from build123d import *
from OCP.BRepFilletAPI import BRepFilletAPI_MakeChamfer

# Parameters (mm, degrees)
SKETCH1_R           = 11.1125
SKETCH1_R_2         = 3.96875
BOSS_EXTRUDE1_DEPTH = 127
CHAMFER1_SIZE       = 0.762
CHAMFER1_SIZE2      = 0.439940905


with BuildPart() as part:
    # Sketch1 → Boss-Extrude1 (new body)
    with BuildSketch(Plane(origin=(0, 0, 0), x_dir=(0, 0, -1), z_dir=(1, 0, 0))):
        Circle(SKETCH1_R)
        Circle(SKETCH1_R_2, mode=Mode.SUBTRACT)
    extrude(amount=BOSS_EXTRUDE1_DEPTH)

    # Chamfer1: one chamfer whose edges measure the first distance from different faces: ONE call of the kernel's chamfer builder (chamfer() names one face for all edges)
    chamfer1_edges_1 = [part.edges().sort_by_distance(p)[0] for p in [
        (0, 0, 11.1125),
    ]]
    chamfer1_side_1 = [part.faces().sort_by_distance(p)[0] for p in [
        (0, 0, 10.798191036),
    ]]
    chamfer1_edges_2 = [part.edges().sort_by_distance(p)[0] for p in [
        (127, 0, 11.1125),
    ]]
    chamfer1_side_2 = [part.faces().sort_by_distance(p)[0] for p in [
        (63.5, 0, 11.1125),
    ]]
    chamfer1_edges_3 = [part.edges().sort_by_distance(p)[0] for p in [
        (0, 0, 3.96875),
    ]]
    chamfer1_side_3 = [part.faces().sort_by_distance(p)[0] for p in [
        (63.5, 0, 3.96875),
    ]]
    chamfer1_edges_4 = [part.edges().sort_by_distance(p)[0] for p in [
        (127, 0, 3.96875),
    ]]
    chamfer1_side_4 = [part.faces().sort_by_distance(p)[0] for p in [
        (127, 0, 10.798191036),
    ]]
    chamfer1 = BRepFilletAPI_MakeChamfer(part.part.solid().wrapped)
    for e in chamfer1_edges_1:
        chamfer1.Add(CHAMFER1_SIZE, CHAMFER1_SIZE2, e.wrapped, chamfer1_side_1[0].wrapped)  # the first distance lies on this face
    for e in chamfer1_edges_2:
        chamfer1.Add(CHAMFER1_SIZE, CHAMFER1_SIZE2, e.wrapped, chamfer1_side_2[0].wrapped)  # the first distance lies on this face
    for e in chamfer1_edges_3:
        chamfer1.Add(CHAMFER1_SIZE, CHAMFER1_SIZE2, e.wrapped, chamfer1_side_3[0].wrapped)  # the first distance lies on this face
    for e in chamfer1_edges_4:
        chamfer1.Add(CHAMFER1_SIZE, CHAMFER1_SIZE2, e.wrapped, chamfer1_side_4[0].wrapped)  # the first distance lies on this face
    add(Compound.cast(chamfer1.Shape()), mode=Mode.REPLACE)


solid = part.part
Build history of the part. All positions in model axes, mm. Round coordinates to 2 decimals unless told otherwise and drop trailing zeros. Loops run counter-clockwise (first coordinate to the right, second up) from the corner with the lowest first, then second, coordinate; pieces in that order, holes last. Notation, with made-up numbers: (13.5, 28) -> (55.5, 28) arc R20 cw to (55.5, 65) -> close; hole circle Ø2 at (81.25, -16). An arc over 180 degrees is marked (long way). Use CSV: the item, a comma, the result in double quotes. Start each with the question number.
Q1. Mould opens along Z. For faces 1 (the face through (127, -2, -5)), 2 (the face through (62.78, -3.874, 0.86)), 3 (the face through (62.46, 3.34, -10.6)) say: +Z half, -Z half, draft (parallel to the pull), parting line (faces both ways), or undercut.
Q2. Flat gauge pins, fed straight in: pin 1 Ø6 at (x, z) = (40, -7.5) entering from -Y; pin 2 Ø3 at (x, y) = (60, 7.5) entering from -Z; pin 3 Ø1.5 at (x, y) = (22.5, -6.5) entering from -Z. Where does each tip first touch, or does it go through?
Q3. Drill centre lines: L1, parallel to Y at x = 35.5, z = 0; L2, parallel to Z at x = 56, y = -0.75; L3, parallel to Y at x = 26, z = -0.5. Where is each one in solid material? Low to high.
Q4. Saw through at A-A on z = 0. Give the cut face in (x, y), and give its area (3 significant figures).
Q5. Saw through at C-C on x = 96. Give the cut face in (y, z) (1 decimal), and give its area (3 significant figures).
Solutions:
1,face 1,"draft"
1,face 2,"undercut"
1,face 3,"parting line"
2,pin 1,"stops at y = -10.16"
2,pin 2,"stops at z = -9.35"
2,pin 3,"stops at z = -9.51"
3,L1,"y = -11.11 to -3.97, 3.97 to 11.11"
3,L2,"z = -11.09 to -3.9, 3.9 to 11.09"
3,L3,"y = -11.1 to -3.94, 3.94 to 11.1"
4,outline,"(0, -10.35) -> (0.44, -11.11) -> (126.24, -11.11) -> (127, -10.67) -> (127, -4.73) -> (126.56, -3.97) -> (0.76, -3.97) -> (0, -4.41) -> close; (0, 4.41) -> (0.76, 3.97) -> (126.56, 3.97) -> (127, 4.73) -> (127, 10.67) -> (126.24, 11.11) -> (0.44, 11.11) -> (0, 10.35) -> close"
4,area,"1,810 mm^2"
5,outline,"circle Ø22.2 at (0, 0); hole circle Ø7.9 at (0, 0)"
5,area,"338 mm^2"
